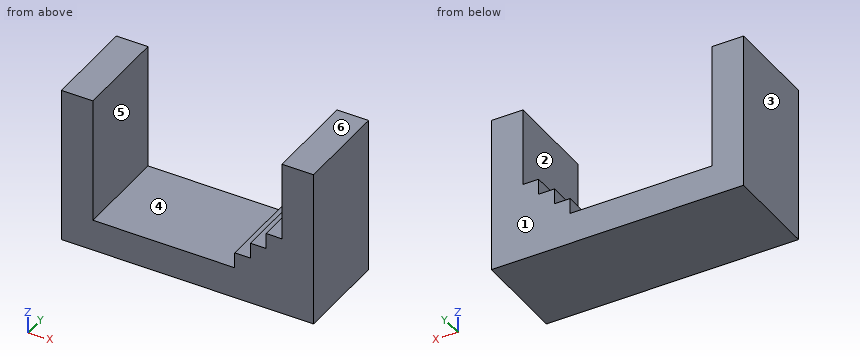
Autodesk Inventor part; units mm, degrees
ref_plane "YZ Plane" through (0, 0, 0) normal (1, 0, 0) x (0, 1, 0)
ref_plane "XZ Plane" through (0, 0, 0) normal (0, 1, 0) x (-1, 0, 0)
ref_plane "XY Plane" through (0, 0, 0) normal (0, 0, 1) x (1, 0, 0)
sketch "Sketch1" plane through (0, 0, 0) normal (0, 1, 0) x (-1, 0, 0)
  line L0 (0, 0) -> (50.8, 0)
  line L1 (50.8, 0) -> (50.8, 31.75)
  line L2 (50.8, 31.75) -> (0, 31.75)
  line L3 (0, 31.75) -> (0, 0)
  line L4 (0, 0) -> (6.35, 0)
  line L5 (6.35, 0) -> (6.35, 6.35)
  line L6 (6.35, 6.35) -> (0, 6.35)
  line L7 (0, 6.35) -> (0, 0)
  line L8 (6.35, 6.35) -> (44.45, 6.35)
  line L9 (44.45, 6.35) -> (44.45, 31.75)
  line L10 (44.45, 31.75) -> (6.35, 31.75)
  line L11 (6.35, 31.75) -> (6.35, 6.35)
  line L12 (6.35, 6.35) -> (12.7, 6.35)
  line L13 (12.7, 6.35) -> (12.7, 12.7)
  line L14 (12.7, 12.7) -> (6.35, 12.7)
  line L15 (6.35, 12.7) -> (6.35, 6.35)
  line L16 (12.7, 6.35) -> (15.875, 6.35)
  line L17 (15.875, 6.35) -> (15.875, 9.525)
  line L18 (15.875, 9.525) -> (12.7, 9.525)
  line L19 (12.7, 9.525) -> (12.7, 6.35)
  line L20 (6.35, 12.7) -> (9.525, 12.7)
  line L21 (9.525, 12.7) -> (9.525, 15.875)
  line L22 (9.525, 15.875) -> (6.35, 15.875)
  line L23 (6.35, 15.875) -> (6.35, 12.7)
  dimension "d0" = 50.8
  dimension "d1" = 31.75
  dimension "d2" = 6.35
  dimension "d3" = 6.35
  dimension "d4" = 38.1
  dimension "d5" = 25.4
  dimension "d6" = 6.35
  dimension "d7" = 6.35
  dimension "d8" = 3.175
  dimension "d9" = 3.175
  dimension "d10" = 3.175
  dimension "d11" = 3.175
extrude "Extrusion1" add sketch "Sketch1" along normal blind 19.05 contours L3 L6 L5 L0 | L5 L8 L9 L2 L1 L0 | L3 L2 L11 L6 | L11 L14 L13 L8 | L13 L18 L17 L8 | L11 L22 L21 L14
properties part number "penHolderHolder"
Design review of the part built by this model. Coordinates are the model's own, in mm. Face numbers are marked on the shaded views. A direction names the side the tool comes from. Round coordinates to 2 decimals unless told otherwise and drop trailing zeros. Write each loop counter-clockwise with the first axis right and the second up, starting at its lowest first coordinate (ties: lowest second). Pieces come first, ordered by that corner, then holes. Notation, with made-up numbers: (7.25, -17) -> (37.25, -17) arc R13 cw to (37.25, 0) -> close; hole circle Ø2 at (24.25, -30). An arc over 180 degrees is marked (long way). Answer in a Markdown table with one row per item.
Q1. Take a section at B-B, the plane z = 18. State the section outline as (x, y) points.
The answers:
| item | result |
|---|---|
| outline | (-50.8, 0) -> (-44.45, 0) -> (-44.45, 19.05) -> (-50.8, 19.05) -> close; (-6.35, 0) -> (0, 0) -> (0, 19.05) -> (-6.35, 19.05) -> close |
Q2. For the marked faces 1 and 2, list the 3-axis set-ups (+Z, -Z, +X, -X, +Y, -Y) from which the entire face can be reached by the end or side of a thin tool; tool diameter is ignored.
The answers:
| item | result |
|---|---|
| face 1 | +Z, -Z, +X, -X, +Y |
| face 2 | +Z, +Y, -Y |
Q3. Take a section at C-C, the plane y = 11.5. State the section outline as (x, z) points (3 decimals), then the cut area to 3 significant figures.
The answers:
| item | result |
|---|---|
| outline | (-50.8, 0) -> (0, 0) -> (0, 31.75) -> (-6.35, 31.75) -> (-6.35, 15.875) -> (-9.525, 15.875) -> (-9.525, 12.7) -> (-12.7, 12.7) -> (-12.7, 9.525) -> (-15.875, 9.525) -> (-15.875, 6.35) -> (-44.45, 6.35) -> (-44.45, 31.75) -> (-50.8, 31.75) -> close |
| area | 706 mm² |
Q4. To check wall thickness, follow L1, parallel to X at y = 1, z = 24; L2, parallel to Z at x = -34.5, y = 11.25; L3, parallel to Z at x = -8, y = 6.5 (3 decimals). State the ranges of each line that lie inside material, in increasing order. Write a range as [from, to].
The answers:
| item | result |
|---|---|
| L1 | [-50.8, -44.45], [-6.35, 0] |
| L2 | [0, 6.35] |
| L3 | [0, 15.875] |
Q5. Clearance check with flat-ended pins moving along their axes: pin 1 Ø9.5 at (x, y) = (-24.5, 12) entering from +Z; pin 2 Ø4 at (x, y) = (-17, 11.5) entering from +Z (3 decimals); pin 3 Ø2.5 at (x, y) = (-11.5, 7) entering from +Z. State where each tip first meets the part, or that it passes through.
The answers:
| item | result |
|---|---|
| pin 1 | z = 6.35 |
| pin 2 | z = 9.525 |
| pin 3 | z = 12.7 |
Q6. Take a section at D-D, the plane x = -38.5. State the section outline as (y, z) points, then the cut area to 3 significant figures.
The answers:
| item | result |
|---|---|
| outline | (0, 0) -> (19.05, 0) -> (19.05, 6.35) -> (0, 6.35) -> close |
| area | 121 mm² |
Q7. Draft analysis for pull direction X (two halves, no side actions). For the marked faces 3, 4, 5 and 6, state which applies: +X half, -X half, draft (parallel to the pull), parting line (faces both ways), or undercut.
The answers:
| item | result |
|---|---|
| face 3 | -X half |
| face 4 | undercut |
| face 5 | undercut |
| face 6 | draft |
Q8. Take a section at A-A, the plane z = 13.5. State the section outline as (x, y) points (3 decimals).
The answers:
| item | result |
|---|---|
| outline | (-50.8, 0) -> (-44.45, 0) -> (-44.45, 19.05) -> (-50.8, 19.05) -> close; (-9.525, 0) -> (0, 0) -> (0, 19.05) -> (-9.525, 19.05) -> close |
